```python
from build123d import *

# Parameters (mm, degrees)
BOSS_EXTRU_1_DEPTH = 10


with BuildPart() as part:
    # Esquisse1 → Boss.-Extru.1 (new body)
    with BuildSketch(Plane.XY):
        Polygon((-10, 17.320508076), (10, 17.320508076), (20, 0), (10, -17.320508076), (-10, -17.320508076), (-20, 0), align=None)
    boss_extru_1 = extrude(amount=BOSS_EXTRU_1_DEPTH)

    # Esquisse2 → Révolution1 (revolve)
    with BuildSketch(Plane(origin=(0, 0, 0), x_dir=(1, 0, 0), z_dir=(0, 1, 0)), mode=Mode.PRIVATE) as r_volution1_sk:
        Polygon((0, -10), (0, -70), (9, -70), (10, -69), (10, -10), align=None)
    r_volution1 = revolve(r_volution1_sk.sketch.rotate(Axis((0, 0, 10), (0, 0, 1)), 180), axis=Axis((0, 0, 10), (0, 0, 1)))

    # Symétrie1: Boss.-Extru.1, Révolution1 across plane
    add(boss_extru_1.mirror(Plane(origin=(0, 0, 0), x_dir=(1, 0, 0), z_dir=(0, 0, -1))))
    add(r_volution1.mirror(Plane(origin=(0, 0, 0), x_dir=(1, 0, 0), z_dir=(0, 0, -1))))


solid = part.part
```
Work out the finished part from the listing and answer in its coordinate system (mm). A direction names the side the tool comes from. Coordinates: 2 decimals unless noted, no trailing zeros. Loops run counter-clockwise (first coordinate to the right, second up) from the corner with the lowest first, then second, coordinate; pieces in that order, holes last. Notation, with made-up numbers: M 53.5,25 L 72.5,25 A32 ccw 72.5,59 Z; hole C -20.75,-37.5 d7. An arc over 180 degrees is marked long. Use CSV: the item, a comma, the result in double quotes. Start each with the question number.
(1) For faces 1 (the face through (-9, 8, 10)), 2 (the face through (0, 0, -70)), 3 (the face through (10, 0, -39)), determine the directions among +Z, -Z, +X, -X, +Y, -Y from which every point of the face is accessible in a straight line to the end or side of a thin tool.
(2) Find section C-C, the plane x = 15. Give the vertices of the cut face in (y, z).
(3) Find section B-B, the plane z = 58. Give the vertices of the cut face in (x, y), then the cut area to 3 significant figures.
(4) Find section A-A, the plane x = 0. Give the vertices of the cut face in (y, z).
(5) Consider line 1 (Z direction, x = -10, y = 12); line 2 (X direction, y = -4.5, z = -44); line 3 (Y direction, x = -7, z = 61.5). Determine where each line is inside the solid, lowest interval first.
(6) Given pin 1 Ø2 at (x, z) = (2.5, 49) entering from -Y; pin 2 Ø10 at (x, z) = (5, 45.5) entering from -Y; pin 3 Ø1.5 at (y, z) = (9.5, -39) entering from +X; pin 4 Ø2 at (y, z) = (-12.5, -14) entering from +X, each flat-ended and moving along its own axis, determine where each tip first touches the part or whether it passes through.
Recorded:
1,face 1,"+Z"
1,face 2,"-Z, +X, -X, +Y, -Y"
1,face 3,"-Z"
2,outline,"M -8.66,-10 L 8.66,-10 L 8.66,10 L -8.66,10 Z"
3,outline,"C 0,0 d20"
3,area,"314 mm^2"
4,outline,"M -17.32,-10 L -10,-10 L -10,-69 L -9,-70 L 9,-70 L 10,-69 L 10,-10 L 17.32,-10 L 17.32,10 L 10,10 L 10,69 L 9,70 L -9,70 L -10,69 L -10,10 L -17.32,10 Z"
5,line 1,"z = -10 to 10"
5,line 2,"x = -8.93 to 8.93"
5,line 3,"y = -7.14 to 7.14"
6,pin 1,"stops at y = -9.89"
6,pin 2,"stops at y = -10"
6,pin 3,"stops at x = 4.84"
6,pin 4,"passes through"
